Autodesk Inventor part; units mm, degrees
ref_plane "YZ Plane" through (0, 0, 0) normal (1, 0, 0) x (0, 1, 0)
ref_plane "XZ Plane" through (0, 0, 0) normal (0, 1, 0) x (-1, 0, 0)
ref_plane "XY Plane" through (0, 0, 0) normal (0, 0, 1) x (1, 0, 0)
sketch "Sketch1" plane through (0, 0, 0) normal (0, 0, 1) x (1, 0, 0)
  line L0 (-23, -24) -> (23, -24)
  line L1 (23, -24) -> (23, 24)
  line L2 (23, 24) -> (-23, 24)
  line L3 (-23, 24) -> (-23, -24)
  line L4 (-23, -24) -> (23, 24) construction
  line L5 (23, -24) -> (-23, 24) construction
  point P0 (0, 0)
  dimension "d0" = 46
  dimension "d1" = 48
extrude "Plate1" add sketch "Sketch1" along normal blind 3
fillet "Corner Round1" radius 4 4 edges at (23, -24, 1.5) (23, 24, 1.5) (-23, -24, 1.5) (-23, 24, 1.5)
sketch "Sketch2" plane through (0, 0, 3) normal (0, 0, 1) x (1, 0, 0)
  circle A0 centre (0, 0) radius 7.25
  dimension "d4" = 14.5
extrude "Extrusion1" cut sketch "Sketch2" against normal through all
equation "\"d2\" = Thickness"
equation "\"BendRadius\" = Thickness"
equation "\"BendReliefWidth\" = Thickness"
equation "\"BendReliefDepth\" = 0.5 * Thickness"
equation "\"CornerReliefSize\" = 4 * Thickness"
equation "\"MinimumRemnant\" = 2 * Thickness"
equation "\"TransitionRadius\" = BendRadius"
equation "\"JacobiRadiusSize\" = BendRadius"
equation "\"GapSize\" = Thickness"
properties part number "NDM 4.0.2  base plate" material "Stainless Steel"
Can you work these out from the model? Positions are in its coordinate system, mm. Round coordinates to 2 decimals unless told otherwise and drop trailing zeros. Loops run counter-clockwise (first coordinate to the right, second up) from the corner with the lowest first, then second, coordinate; pieces in that order, holes last. Notation, with made-up numbers: M 52,65 L 98,65 A29 cw 98,99 Z; hole C -40,67 d5. An arc over 180 degrees is marked long. Answer in a Markdown table with one row per item.
1. If we section it at A-A, the plane x = 0: Please give me the cut outline in (y, z), plus the area to 4 significant figures.
Established:
| item | result |
|---|---|
| outline | M -24,0 L -7.25,0 L -7.25,3 L -24,3 Z; M 7.25,0 L 24,0 L 24,3 L 7.25,3 Z |
| area | 100.5 mm² |
2. Please list where these lines run through material, in increasing order: line 1 (Y direction, x = 0, z = 1.5); line 2 (Y direction, x = -3, z = 2.25); line 3 (X direction, y = -2, z = 2.95). Write a range as from..to.
Established:
| item | result |
|---|---|
| line 1 | -24..-7.25, 7.25..24 |
| line 2 | -24..-6.6, 6.6..24 |
| line 3 | -23..-6.97, 6.97..23 |
3. If we section it at B-B, the plane y = 0: Please give me the cut outline in (x, z), plus the area to 3 significant figures.
Established:
| item | result |
|---|---|
| outline | M -23,0 L -7.25,0 L -7.25,3 L -23,3 Z; M 7.25,0 L 23,0 L 23,3 L 7.25,3 Z |
| area | 94.5 mm² |
4. If we section it at C-C, the plane z = 0.55: Please give me the cut outline in (x, y).
Established:
| item | result |
|---|---|
| outline | M -23,-20 A4 ccw -19,-24 L 19,-24 A4 ccw 23,-20 L 23,20 A4 ccw 19,24 L -19,24 A4 ccw -23,20 Z; hole C 0,0 d14.5 |
5. I'm going to push a flat-ended pin straight in: pin 1 Ø12 at (x, y) = (-16.5, -6.5) entering from -Z. Where does the tip first touch, or does it pass through?
Established:
| item | result |
|---|---|
| pin 1 | z = 0 |
6. Thinking about a two-plate mould opening in X: for faces 1 (the face through (-5, 6, 0)), 2 (the face through (-21.797, 22.859, 1.521)), 3 (the face through (3.35, -6.43, 1.52)), which applies, pulls with the +X half, pulls with the -X half, needs draft (parallel to the pull), parting line crosses it, or undercut?
Established:
| item | result |
|---|---|
| face 1 | needs draft |
| face 2 | pulls with the -X half |
| face 3 | undercut |
